Autodesk Inventor part; units mm, degrees
ref_plane "YZ Plane" through (0, 0, 0) normal (1, 0, 0) x (0, 1, 0)
ref_plane "XZ Plane" through (0, 0, 0) normal (0, 1, 0) x (-1, 0, 0)
ref_plane "XY Plane" through (0, 0, 0) normal (0, 0, 1) x (1, 0, 0)
sketch "Sketch1" plane through (0, 0, 0) normal (0, 0, 1) x (1, 0, 0)
  line L0 (0, 0) -> (130.048, 0)
  line L1 (87.9024, 12.7) -> (59.6729, 12.7)
  line L2 (87.9024, 12.7) -> (130.048, 12.7)
  line L3 (130.048, 12.7) -> (130.048, 0)
  line L4 (130.048, -25.4) -> (142.748, -25.4)
  line L5 (130.048, -25.4) -> (144.7127, 0)
  line L6 (142.748, -25.4) -> (164.745, 12.7)
  line L7 (144.7127, 0) -> (130.048, 0)
  line L8 (130.048, 12.7) -> (164.745, 12.7)
  line L9 (0, 0) -> (7.3323, 12.7)
  line L10 (3.6662, 6.35) -> (20.4175, 35.3641)
  line L11 (3.6662, 6.35) -> (-13.0851, -22.6641)
  line L12 (-13.0851, -22.6641) -> (-78.9003, 15.3343)
  line L13 (-78.9003, 15.3343) -> (-45.3977, 73.3625)
  line L14 (-45.3977, 73.3625) -> (20.4175, 35.3641)
  line L15 (20.4175, 35.3641) -> (59.6729, 12.7)
  line L16 (20.4175, 35.3641) -> (13.4893, 39.3641)
  circle A0 centre (6.7393, 27.6728) radius 4.15
  line L17 (-78.9003, 15.3343) -> (-71.9721, 11.3343)
  circle A1 centre (-65.2221, 23.0256) radius 4.1529
  line L18 (-45.3977, 73.3625) -> (-38.4686, 69.362)
  circle A2 centre (-45.2174, 57.6728) radius 4.1529
  line L19 (-13.0851, -22.6641) -> (-6.3414, -10.9837)
  line L20 (-6.3414, -10.9837) -> (-13.2705, -6.9832)
  circle A3 centre (-13.2705, -6.9832) radius 4.0259
  dimension "d39" = 130.048
  dimension "d41" = 25.4
  dimension "d42" = 12.7
  dimension "d43" = 60
  dimension "d44" = 60
  dimension "d45" = 12.7
  dimension "d51" = 136.3234
  dimension "d54" = 136.3234
  dimension "d55" = 12.7
  dimension "d56" = 66.5476
  dimension "d57" = 33.5026
  dimension "d58" = 33.5026
  dimension "d59" = 75.9968
  dimension "d60" = 40.8349
  dimension "d61" = 8
  dimension "d63" = 8.3
  dimension "d64" = 8
  dimension "d66" = 8.3058
  dimension "d69" = 8.001
  dimension "d70" = 13.5
  dimension "d72" = 8.3058
  dimension "d73" = 13.4874
  dimension "d74" = 8.001
  dimension "d75" = 90
  dimension "d76" = 8.0518
extrude "Extrusion2" add sketch "Sketch1" along normal blind 6.35
properties part number "hook" material "Steel"
Verification items for the finished model (mm, model axes). A direction names the side the tool comes from. Coordinates: 2 decimals unless noted, no trailing zeros. Write each loop counter-clockwise with the first axis right and the second up, starting at its lowest first coordinate (ties: lowest second). Pieces come first, ordered by that corner, then holes. Notation, with made-up numbers: M 54,43 L 93,43 A28 ccw 93,70 Z; hole C 51,-4 d5. An arc over 180 degrees is marked long. One line per item, written item: value.
Item 1: Section check B-B, the plane z = 3.75. State how many separate pieces and enclosed holes the cut face has, plus the area to 3 significant figures.
Check sheet entries:
separate pieces: 1
enclosed holes: 4
area: 7,790 mm^2
Item 2: Section check A-A, the plane y = -19. Record the boundary of the cut face in (x, z), plus the area to 3 significant figures.
Check sheet entries:
outline: M -19.43,0 L -10.97,0 L -10.97,6.35 L -19.43,6.35 Z; M 133.74,0 L 146.44,0 L 146.44,6.35 L 133.74,6.35 Z
area: 134 mm^2
Item 3: Gauge pin test, flat ends, axial feed: pin 1 Ø1 at (x, z) = (-40.5, 2) entering from +Y; pin 2 Ø1.9 at (x, z) = (94, 3) entering from +Y; pin 3 Ø1 at (y, z) = (29.5, 0.5) entering from -X. Record the tip position at first contact, or that the pin passes through.
Check sheet entries:
pin 1: stops at y = 70.82
pin 2: stops at y = 12.7
pin 3: stops at x = -71.01
Item 4: Section check C-C, the plane x = 124. Record the boundary of the cut face in (y, z), plus the area to 3 significant figures.
Check sheet entries:
outline: M 0,0 L 12.7,0 L 12.7,6.35 L 0,6.35 Z
area: 80.6 mm^2
Item 5: Mould release check, pull along X, two halves, no side actions. Record for faces 4 (the flat face through (-45.53, -3.93, 3.13)), 5 (the flat face through (113, 12.7, 3)), 6 (the cylindrical face through (5.84, 31.724, 3.131)): pulls with the +X half, pulls with the -X half, needs draft (parallel to the pull), parting line crosses it, or undercut.
Check sheet entries:
face 4: pulls with the -X half
face 5: needs draft
face 6: undercut
Item 6: Access from +Z, -Z, +X, -X, +Y, -Y to the whole of each face (thin tool, end or side, straight path). Record for faces 1 (the flat face through (-6.45, -11.17, 3.13)), 2 (the flat face through (6, 13, 6.35)), 3 (the flat face through (137.278, -12.878, 3.131)).
Check sheet entries:
face 1: +Z, -Z, -Y
face 2: +Z, +X, -X, +Y, -Y
face 3: +Z, -Z
Item 7: Scan lines: line 1 along Y through (x, z) = (71, 1.25); line 2 along X through (y, z) = (-10.5, 3.5); line 3 along Y through (x, z) = (6.5, 2). Record each from-to range of solid material in increasing order.
Check sheet entries:
line 1: y = 0 to 12.7
line 2: x = -34.15 to -15.23, -11.31 to -6.06, 138.65 to 151.35
line 3: y = 0 to 23.53, 31.82 to 43.4
Item 8: Section check D-D, the plane y = 39. Record the boundary of the cut face in (x, z), plus the area to 3 significant figures.
Check sheet entries:
outline: M -65.24,0 L 14.12,0 L 14.12,6.35 L -65.24,6.35 Z
area: 504 mm^2
